from build123d import *

# Parameters (mm, degrees)
SKETCH2_W           = 31.9
SKETCH2_H           = 43.46
BOSS_EXTRUDE1_DEPTH = 16.94
SHELL1_T            = -1.6
SKETCH3_W           = 5
SKETCH3_H           = 1
BOSS_EXTRUDE2_DEPTH = 1
SKETCH4_W           = 5
SKETCH4_H           = 1
BOSS_EXTRUDE3_DEPTH = 1
CHAMFER1_SIZE       = 1
CUT_EXTRUDE1_DEPTH  = 32.014690068


with BuildPart() as part:
    # Sketch2 → Boss-Extrude1 (new body)
    with BuildSketch(Plane(origin=(0, 0, 0), x_dir=(0, 1, 0), z_dir=(0, 0, 1))):
        Rectangle(SKETCH2_W, SKETCH2_H)
    extrude(amount=BOSS_EXTRUDE1_DEPTH)

    # Shell1
    shell1_openings = [part.faces().sort_by_distance(p)[0] for p in [
        (0, 0, 16.94),
    ]]
    offset(amount=SHELL1_T, openings=shell1_openings, kind=Kind.INTERSECTION)

    # Sketch3 → Boss-Extrude2 (add)
    with BuildSketch(Plane(origin=(0, -14.35, 0), x_dir=(-1, 0, 0), z_dir=(0, 1, 0))):
        with Locations((-12.63, 15.84)):
            Rectangle(SKETCH3_W, SKETCH3_H)
        with Locations((12.63, 15.84)):
            Rectangle(SKETCH3_W, SKETCH3_H)
    extrude(amount=BOSS_EXTRUDE2_DEPTH)

    # Sketch4 → Boss-Extrude3 (add)
    with BuildSketch(Plane.XZ.offset(-14.35)):
        with Locations((-12.63, 15.84)):
            Rectangle(SKETCH4_W, SKETCH4_H)
        with Locations((12.63, 15.84)):
            Rectangle(SKETCH4_W, SKETCH4_H)
    extrude(amount=BOSS_EXTRUDE3_DEPTH)

    # Chamfer1
    chamfer1_edges = [part.edges().sort_by_distance(p)[0] for p in [
        (-12.63, -13.35, 16.34),
        (12.63, -13.35, 16.34),
        (-12.63, 13.35, 16.34),
        (12.63, 13.35, 16.34),
    ]]
    chamfer(chamfer1_edges, length=CHAMFER1_SIZE - 0.0001)  # a hair under: the kernel refuses the full size

    # Sketch5 → Cut-Extrude1 (cut, through all)
    with BuildSketch(Plane.XY.offset(1.6)):
        with BuildLine():
            Line((-20.13, 5), (-20.13, -5))
            ThreePointArc((-20.13, -5), (-15.13, 0), (-20.13, 5))
        make_face()
    extrude(amount=-CUT_EXTRUDE1_DEPTH, mode=Mode.SUBTRACT)


solid = part.part
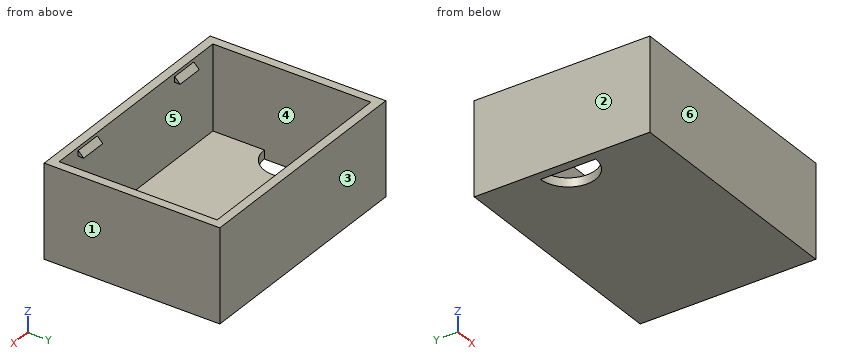
Here's how the part is built. I have some questions about the finished solid (model axes, mm). Face numbers are marked on the shaded views. A direction names the side the tool comes from. Give positions to 0.01 mm unless a question says otherwise; leave off trailing zeros. Order: outer loops, then holes, each group sorted by start corner. A loop starts at its lowest first (then second) coordinate and runs counter-clockwise, first axis right, second up. Notation, with made-up numbers: (39.5, 57) -> (58.5, 57) arc R15 ccw to (58.5, 77) -> close; hole circle Ø6 at (89.5, 64.25). An arc over 180 degrees is marked (long way). One line per item, written item: value. Start each with the question number.
1. For the marked faces 5 and 6, which set-ups out of +Z, -Z, +X, -X, +Y, -Y let a thin tool reach every point of the face, with its end or its side?
2. I need wall thicknesses on probe 1 along Y at (x, z) = (-5, 11.75); probe 2 along X at (y, z) = (4.5, 10.5); probe 3 along Z at (x, y) = (16.5, 5). Which ranges of each line are inside material? Lowest first, please. Write a range as from..to.
3. Imagine slicing it at C-C, the plane x = -18. List the corners of the cut face in (y, z) for me, plus the area to 3 significant figures.
4. Imagine slicing it at B-B, the plane z = 12.75. List the corners of the cut face in (x, y) for me, plus the area to 3 significant figures.
5. Imagine slicing it at D-D, the plane y = -10. List the corners of the cut face in (x, z) for me, plus the area to 3 significant figures.
6. Will this pin go through, and if not, where does the flat tip stop? pin 1 Ø4 at (x, y) = (11.5, 3.5) entering from +Z.
7. We'd pull the mould along X, two halves only. Please class the marked faces 1, 2, 3 and 4: released by +X, released by -X, zero draft, split by the parting line, or undercut.
8. Imagine slicing it at A-A, the plane y = 0. List the corners of the cut face in (x, z) for me.
Values follow:
1. face 5: none
1. face 6: +Z, -Z, +X, -X, -Y
2. probe 1: y = -15.95..-14.35, 14.35..15.95
2. probe 2: x = -21.73..-20.13, 20.13..21.73
2. probe 3: z = 0..1.6
3. outline: (-15.95, 0) -> (-4.52, 0) -> (-4.52, 1.6) -> (-14.35, 1.6) -> (-14.35, 16.94) -> (-15.95, 16.94) -> close; (4.52, 0) -> (15.95, 0) -> (15.95, 16.94) -> (14.35, 16.94) -> (14.35, 1.6) -> (4.52, 1.6) -> close
3. area: 85.7 mm2
4. outline: (-21.73, -15.95) -> (21.73, -15.95) -> (21.73, 15.95) -> (-21.73, 15.95) -> close; hole (-20.13, -14.35) -> (20.13, -14.35) -> (20.13, 14.35) -> (-20.13, 14.35) -> close
4. area: 231 mm2
5. outline: (-21.73, 0) -> (21.73, 0) -> (21.73, 16.94) -> (20.13, 16.94) -> (20.13, 1.6) -> (-20.13, 1.6) -> (-20.13, 16.94) -> (-21.73, 16.94) -> close
5. area: 119 mm2
6. pin 1: stops at z = 1.6
7. face 1: released by +X
7. face 2: released by -X
7. face 3: zero draft
7. face 4: undercut
8. outline: (-21.73, 0) -> (-20.13, 0) -> (-20.13, 16.94) -> (-21.73, 16.94) -> close; (-15.13, 0) -> (21.73, 0) -> (21.73, 16.94) -> (20.13, 16.94) -> (20.13, 1.6) -> (-15.13, 1.6) -> close
